```python
from build123d import *

# Parameters (mm, degrees)
F0_R      = 0.75
F1_DEPTH  = 2
F4_DEPTH  = 11.48
F6_DEPTH  = 11.48
F8_DEPTH  = 11.48
F9_R      = 0.75
F10_DEPTH = 25
F11_R     = 0.75
F12_DEPTH = 25
F13_R     = 0.75
F14_DEPTH = 25


with BuildPart() as f1:
    # F0 (on Top) → F1 (new body)
    with BuildSketch(Plane.XY):
        with BuildLine():
            Line((-31.5357583467, 23.4181724987), (-13.8580888171, 5.7405029691))
            ThreePointArc((-13.8580888171, 5.7405029691), (0, -15), (13.8580888171, 5.7405029691))
            Line((13.8580888171, 5.7405029691), (31.5357583467, 23.4181724987))
            ThreePointArc((31.5357583467, 23.4181724987), (31.5357583467, 31.5357583467), (23.4181724987, 31.5357583467))
            Line((23.4181724987, 31.5357583467), (5.7405029691, 13.8580888171))
            Line((5.7405029691, 13.8580888171), (5.7405029691, 38.8580888171))
            ThreePointArc((5.7405029691, 38.8580888171), (0.0002514811, 44.5983403026), (-5.7400000019, 38.858088812))
            Line((-5.7400000019, 38.858088812), (-5.7405029691, 13.8580888171))
            Line((-5.7405029691, 13.8580888171), (-23.4181724987, 31.5357583467))
            ThreePointArc((-23.4181724987, 31.5357583467), (-31.5357583467, 31.5357583467), (-31.5357583467, 23.4181724987))
        make_face()
        with Locations((-31.5357583467, 27.4769654227)):
            Circle(F0_R, mode=Mode.SUBTRACT)
        with Locations((-27.4769654227, 31.5357583467)):
            Circle(F0_R, mode=Mode.SUBTRACT)
        with Locations((-2.8698742604, 41.7282145573)):
            Circle(F0_R, mode=Mode.SUBTRACT)
        with Locations((31.5357583467, 27.4769654227)):
            Circle(F0_R, mode=Mode.SUBTRACT)
        with Locations((2.8703772251, 41.7282145598)):
            Circle(F0_R, mode=Mode.SUBTRACT)
        with Locations((27.4769654227, 31.5357583467)):
            Circle(F0_R, mode=Mode.SUBTRACT)
    extrude(amount=F1_DEPTH)

    # F3 (on face) → F4 (join)
    with BuildSketch(Plane(origin=(-4.058792924, 4.058792924, 0), x_dir=(0.7071067812, 0.7071067812, 0), z_dir=(0.7071067812, -0.7071067812, 0))):
        Polygon((35.8582971537, 2), (38.8582971537, 2), (38.8582971537, 6), align=None)
        Polygon((31.691630487, 2), (34.691630487, 2), (34.691630487, 6), align=None)
        Polygon((27.5249638204, 2), (30.5249638204, 2), (30.5249638204, 6), align=None)
        Polygon((23.3582971537, 2), (26.3582971537, 2), (26.3582971537, 6), align=None)
        Polygon((19.191630487, 2), (22.191630487, 2), (22.191630487, 6), align=None)
        Polygon((15.0249638204, 2), (18.0249638204, 2), (18.0249638204, 6), align=None)
    extrude(amount=F4_DEPTH)

    # F5 (on face) → F6 (join)
    with BuildSketch(Plane(origin=(-5.7407817733, 0.000115497, 0), x_dir=(-2.01187e-05, -0.9999999998, 0), z_dir=(-0.9999999998, 2.01187e-05, 0))):
        Polygon((-38.8579733229, 6), (-38.8579733229, 2), (-35.8579733229, 2), align=None)
        Polygon((-34.6913066562, 6), (-34.6913066562, 2), (-31.6913066562, 2), align=None)
        Polygon((-30.5246399896, 6), (-30.5246399896, 2), (-27.5246399896, 2), align=None)
        Polygon((-26.3579733229, 6), (-26.3579733229, 2), (-23.3579733229, 2), align=None)
        Polygon((-22.1913066562, 6), (-22.1913066562, 2), (-19.1913066562, 2), align=None)
        Polygon((-18.0246399896, 6), (-18.0246399896, 2), (-15.0246399896, 2), align=None)
    extrude(amount=-F6_DEPTH)

    # F7 (on face) → F8 (join)
    with BuildSketch(Plane(origin=(-4.058792924, -4.058792924, 0), x_dir=(0.7071067812, -0.7071067812, 0), z_dir=(-0.7071067812, -0.7071067812, 0))):
        Polygon((-38.8582971537, 6), (-38.8582971537, 2), (-35.8582971537, 2), align=None)
        Polygon((-31.691630487, 2), (-34.691630487, 6), (-34.691630487, 2), align=None)
        Polygon((-27.5249638204, 2), (-30.5249638204, 6), (-30.5249638204, 2), align=None)
        Polygon((-23.3582971537, 2), (-26.3582971537, 6), (-26.3582971537, 2), align=None)
        Polygon((-19.191630487, 2), (-22.191630487, 6), (-22.191630487, 2), align=None)
        Polygon((-15.0249638204, 2), (-18.0249638204, 6), (-18.0249638204, 2), align=None)
    extrude(amount=-F8_DEPTH)

    # F9 (on face) → F10 (cut)
    with BuildSketch(Plane(origin=(-27.4769654227, 27.4769654227, 0), x_dir=(-0.7071067812, -0.7071067812, 0), z_dir=(-0.7071067812, 0.7071067812, 0))):
        with Locations((0, 4)):
            Circle(F9_R)
    extrude(amount=-F10_DEPTH, mode=Mode.SUBTRACT)

    # F11 (on face) → F12 (cut)
    with BuildSketch(Plane(origin=(0.0007817714, 38.857973315, 0), x_dir=(-0.9999999998, 2.01187e-05, 0), z_dir=(2.01187e-05, 0.9999999998, 0))):
        with Locations((0.0007817745, 4)):
            Circle(F11_R)
    extrude(amount=-F12_DEPTH, mode=Mode.SUBTRACT)

    # F13 (on face) → F14 (cut)
    with BuildSketch(Plane(origin=(27.4769654227, 27.4769654227, 0), x_dir=(-0.7071067812, 0.7071067812, 0), z_dir=(0.7071067812, 0.7071067812, 0))):
        with Locations((0, 4)):
            Circle(F13_R)
    extrude(amount=-F14_DEPTH, mode=Mode.SUBTRACT)


solid = f1.part
```
The listing builds one solid part. Answer for the finished solid, in the listing's coordinates (mm). A direction names the side the tool comes from. Round coordinates to 2 decimals unless told otherwise and drop trailing zeros. Write each loop counter-clockwise with the first axis right and the second up, starting at its lowest first coordinate (ties: lowest second). Pieces come first, ordered by that corner, then holes. Notation, with made-up numbers: (-28.75, -22.5) -> (-14.75, -22.5) arc R25 ccw to (-14.75, -5.5) -> close; hole circle Ø10 at (36, 84.25). An arc over 180 degrees is marked (long way). Write item = value, one per line.
1) Section B-B on y = 0 is taken. Write down the section's boundary in (x, z).
Check values:
outline = (-15, 0) -> (15, 0) -> (15, 2) -> (-15, 2) -> close
2) Which of the six approach directions +Z, -Z, +X, -X, +Y, -Y give full straight-line access (tool end or side, diameter ignored) to faces 1 (the flat face through (27.42, 27.534, 3.083)), 2 (the cylindrical face through (30.94, 27.02, 0.99)), 3 (the flat face through (-20.09, 19.98, 3.08)), 4 (the flat face through (-27.534, 27.42, 4.917))?
Check values:
face_1 = +Z, +X, +Y
face_2 = +Z, -Z
face_3 = +Z
face_4 = +Z, -X, +Y
3) Section A-A on z = 0.75 is taken. Write down the section's boundary in (x, y), plus the area to 3 significant figures.
Check values:
outline = (-31.54, 23.42) -> (-13.86, 5.74) arc R15 ccw (long way) to (13.86, 5.74) -> (31.54, 23.42) arc R5.74 ccw to (23.42, 31.54) -> (5.74, 13.86) -> (5.74, 38.86) arc R5.74 ccw to (-5.74, 38.86) -> (-5.74, 13.86) -> (-23.42, 31.54) arc R5.74 ccw to start; hole circle Ø1.5 at (-31.54, 27.48); hole circle Ø1.5 at (-27.48, 31.54); hole circle Ø1.5 at (-2.87, 41.73); hole circle Ø1.5 at (2.87, 41.73); hole circle Ø1.5 at (27.48, 31.54); hole circle Ø1.5 at (31.54, 27.48)
area = 1,690 mm²
4) Straight lines are drawn through the part: line 1 along Y through (x, z) = (4.5, 3.7); line 2 along Y through (x, z) = (24, 2.4); line 3 along Y through (x, z) = (14, 3.25). For each, find the intervals that lie inside material, in ascending order. Write a range as [from, to].
Check values:
line_1 = [16.3, 18.02], [20.47, 22.19], [24.63, 26.36], [28.8, 30.52], [32.97, 34.69], [37.13, 38.86]
line_2 = [15.88, 19.17], [21.24, 25.06], [27.14, 30.95]
line_3 = [8.57, 11.49], [14.47, 17.38], [20.36, 22.12]
5) Section C-C on x = 0 is taken. Give the number of separate pieces and of enclosed holes in the cut face, plus the area to 3 significant figures.
Check values:
separate_pieces = 7
enclosed_holes = 0
area = 142 mm²
6) Given pin 1 (1.5 mm diameter, centred on y = 37, z = 4, fed in from +X); pin 2 (4.5 mm diameter, centred on x = 25.5, y = 25.5, fed in from +Z); pin 3 (1.7 mm diameter, centred on x = 0, z = 4, fed in from -Y); pin 4 (12 mm diameter, centred on x = -13.5, y = 9.5, fed in from -Z), each flat-ended and moving along its own axis, determine where each tip first touches the part or whether it passes through.
Check values:
pin_1 = 5.74
pin_2 = 6
pin_3 = 15.89
pin_4 = 0
7) For a pull along Z with two mould halves and no side action, classify faces 5 (the flat face through (18.581, 18.695, 3.083)), 6 (the flat face through (20.95, 21.07, 4.92)), 7 (the cylindrical face through (0.162, 33.86, 3.268)) as released by +Z, released by -Z, zero draft, split by the parting line, or undercut.
Check values:
face_5 = zero draft
face_6 = released by +Z
face_7 = undercut
